from build123d import *

# Parameters (mm, degrees)
BOSS_EXTRUDE1_DEPTH = 4
SKETCH1_3_R         = 10
CUT_EXTRUDE2_DEPTH  = 19.5
CUT_EXTRUDE3_DEPTH  = 59.5
FILLET2_R           = 2
FILLET9_R           = 2
FILLET10_R          = 1


with BuildPart() as part:
    # Sketch1 → Boss-Extrude1 (new body)
    with BuildSketch(Plane.XY):
        with BuildLine():
            Line((-24.953935647, 1.516936291), (-31.175265199, -100.825303282))
            ThreePointArc((-31.175265199, -100.825303282), (-52.615931746, -148.5955614), (-100.637442791, -169.467413729))
            Line((-100.637442791, -169.467413729), (-107.049597612, -186.395076324))
            ThreePointArc((-107.049597612, -186.395076324), (-31.236424704, -167.329888663), (12.223577372, -102.350301202))
            Line((12.223577372, -102.350301202), (24.801457775, -3.144470101))
            ThreePointArc((24.801457775, -3.144470101), (2.331949777, 24.891002596), (-24.953935647, 1.516936291))
        make_face()
    extrude(amount=BOSS_EXTRUDE1_DEPTH)

    # Sketch1<3> → Cut-Extrude2 (cut)
    with BuildSketch(Plane.XY):
        Circle(SKETCH1_3_R)
    extrude(amount=CUT_EXTRUDE2_DEPTH, mode=Mode.SUBTRACT)

    # Sketch1<4> → Cut-Extrude3 (cut)
    with BuildSketch(Plane.XY):
        Polygon((6.347009132, -61.537145709), (-13.655055469, -72.161869066), (0.810016745, -99.393760114), align=None)
        Polygon((-21.064699943, -77.437028338), (-6.079431787, -105.648238327), (-21.064699943, -113.608133056), align=None)
        Polygon((-26.234337885, -155.650813652), (-46.824530665, -155.650813652), (-57.99672275, -173.202762284), align=None)
        Polygon((-59.711910653, -163.410469366), (-69.148377202, -178.235525617), (-87.829466791, -178.235525617), align=None)
        Polygon((-26.234337885, -126.17530166), (-24.953935647, -148.446836425), (-41.663691875, -148.446836425), align=None)
        Polygon((-18.747269764, -122.305223747), (-2.374159237, -113.608133056), (-17.707255347, -140.395411768), align=None)
        Polygon((-17.949592316, -63.337916036), (7.016311499, -48.830036106), (-15.620624799, -29.988511388), align=None)
    extrude(amount=CUT_EXTRUDE3_DEPTH, mode=Mode.SUBTRACT)

    # Fillet2
    fillet2_edges = [part.edges().sort_by_distance(p)[0] for p in [
        (-15.620624799, -29.988511388, 2),
        (-17.949592316, -63.337916036, 2),
        (7.016311499, -48.830036106, 2),
        (-21.064699943, -77.437028338, 2),
        (-21.064699943, -113.608133056, 2),
        (-6.079431787, -105.648238327, 2),
        (0.810016745, -99.393760114, 2),
        (6.347009132, -61.537145709, 2),
        (-13.655055469, -72.161869066, 2),
    ]]
    fillet(fillet2_edges, radius=FILLET2_R)

    # Fillet9
    fillet9_edges = [part.edges().sort_by_distance(p)[0] for p in [
        (-18.747269764, -122.305223747, 2),
        (-24.953935647, -148.446836425, 2),
        (-46.824530665, -155.650813652, 2),
        (-69.148377202, -178.235525617, 2),
    ]]
    fillet(fillet9_edges, radius=FILLET9_R)

    # Fillet10
    fillet10_edges = [part.edges().sort_by_distance(p)[0] for p in [
        (-17.707255347, -140.395411768, 2),
        (-2.374159237, -113.608133056, 2),
        (-26.234337885, -126.17530166, 2),
        (-41.663691875, -148.446836425, 2),
        (-57.99672275, -173.202762284, 2),
        (-26.234337885, -155.650813652, 2),
        (-87.829466791, -178.235525617, 2),
        (-59.711910653, -163.410469366, 2),
    ]]
    fillet(fillet10_edges, radius=FILLET10_R)


solid = part.part
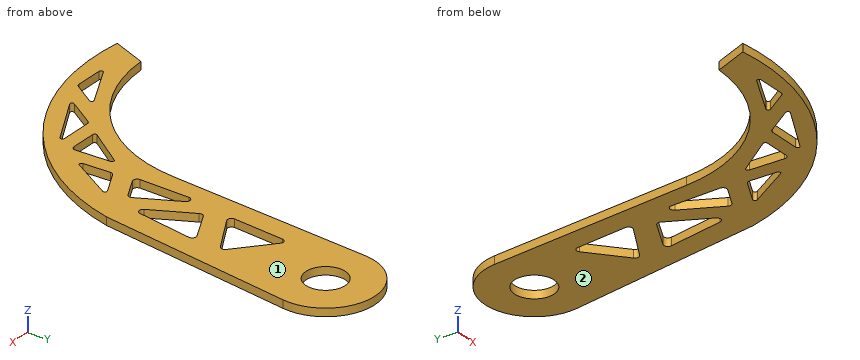
Geometry: final body of the model. Coordinates: model frame, mm. Face numbers are marked on the shaded views. Give positions to 0.01 mm unless a question says otherwise; leave off trailing zeros. Loops run counter-clockwise (first coordinate to the right, second up) from the corner with the lowest first, then second, coordinate; pieces in that order, holes last. Notation, with made-up numbers: M 77.5,83.25 L 101.5,83.25 A14 ccw 101.5,107.25 Z; hole C 37.5,56.25 d9. An arc over 180 degrees is marked long. Put each result on its own line as item: value.
1) Material intervals for L1, parallel to Y at x = 0, z = 2.15; L2, parallel to X at y = 0, z = 1.2; L3, parallel to X at y = -88, z = 1.45, sorted ascending. Write a range as from..to.
Computed values:
L1: y = -133.34..-95.05, -64.91..-52.91, -42.99..-10, 10..25
L2: x = -25.05..-10, 10..25
L3: x = -30.4..-21.06, -15.45..-5.24, 2.48..14.04
2) Mould query, pull axis Z, two halves, no side actions, for the marked faces 1 and 2. Classes: released by +Z, released by -Z, zero draft, split by the parting line, or undercut.
Computed values:
face 1: released by +Z
face 2: released by -Z
3) Cut plane C-C, the plane z = 3.1. Give the number of separate pieces and of enclosed holes in the cut face, plus the area to 3 significant figures.
Computed values:
separate pieces: 1
enclosed holes: 8
area: 7,630 mm^2
4) Cut plane B-B, the plane x = -43. Return the cut outline in (y, z), plus the area to 3 significant figures.
Computed values:
outline: M -174.55,0 L -164.92,0 L -164.92,4 L -174.55,4 Z; M -155.65,0 L -136.86,0 L -136.86,4 L -155.65,4 Z
area: 114 mm^2
5) First-contact query: P1, Ø2, axis at x = -79, z = 1, coming from the +Y side; P2, Ø1.2, axis at x = -40, z = 2.5, coming from the -Y side. Flat tips, straight axial feed; report the tip coordinate or a pass-through.
Computed values:
P1: stops at y = -164.87
P2: stops at y = -173.24
6) Cut plane A-A, the plane y = -6. Return the cut outline in (x, z), plus the area to 3 significant figures.
Computed values:
outline: M -25.41,0 L -8,0 L -8,4 L -25.41,4 Z; M 8,0 L 24.44,0 L 24.44,4 L 8,4 Z
area: 135 mm^2
